Geometry check sheet. Reference: the model listing, model coordinates, mm. A direction names the side the tool comes from. Round coordinates to 2 decimals unless told otherwise and drop trailing zeros. Order: outer loops, then holes, each group sorted by start corner. A loop starts at its lowest first (then second) coordinate and runs counter-clockwise, first axis right, second up. Notation, with made-up numbers: (53, 22) -> (111, 22) arc R12 cw to (111, 37) -> close; hole circle Ø9 at (-4.75, 57.25). An arc over 180 degrees is marked (long way). Use a Markdown table: item, result. Add a question column.
Item 1: Sectioned sample at D-D, the plane x = -43. Record the cut outline in (y, z), and give its area (3 significant figures).
Item 2: Set-up check for faces 1 (the flat face through (-2, -28, -32.703)), 2 (the flat face through (-47.067, -29, 8)): record each of +Z, -Z, +X, -X, +Y, -Y from which the full face is reachable in a straight line by a thin tool's end or side.
Item 3: Gauge pin test, flat ends, axial feed: pin 1 Ø10 at (x, z) = (-10.5, -6.5) entering from +Y; pin 2 Ø2 at (x, z) = (1, 13) entering from -Y. Record the tip position at first contact, or that the pin passes through.
Item 4: Sectioned sample at B-B, the plane z = 6.5. Record the cut outline in (x, y), and give its area (3 significant figures).
Item 5: Mould release check, pull along Y, two halves, no side actions. Record for faces 3 (the flat face through (0, 0, 8)), 4 (the flat face through (-49.567, -28, 8)), 5 (the flat face through (0, -2.5, 8)), 6 (the cylindrical face through (-0.626, -25.635, 46.686)): pulls with the +Y half, pulls with the -Y half, needs draft (parallel to the pull), parting line crosses it, or undercut.
Item 6: Sectioned sample at A-A, the plane y = -18. Record the cut outline in (x, z).
Item 7: Material ranges on probe 1 along Z at (x, y) = (-16.5, -36); probe 2 along X at (y, z) = (-5.5, 13.5); probe 3 along Y at (x, z) = (-37, -23.5), recorded low to high. Write a range as [from, to].
Item 8: Sectioned sample at C-C, the plane x = -13.5. Record the cut outline in (y, z), and give its area (3 significant figures).
from build123d import *

# Parameters (mm, degrees)
F3_T     = -2.5
F5_D     = 30
F5_DEPTH = 12
F5_TIP   = 9.0129092854


with BuildPart() as f2:
    # F2: sweep along a path in F1
    with BuildLine(Plane.YZ) as f2_path:
        Line((0, 0), (-55.432960391, 0))
    # F0 (on Front) → F2 (sweep)
    with BuildSketch(Plane.XZ):
        Polygon((-49.567040056, 47.953914851), (-49.567040056, 42.0879907906), (-49.567040056, -32.7025167644), (47.8072650731, -32.7025167644), (47.8072650731, 47.953914851), align=None)
    sweep(path=f2_path.line)

    # F3
    f3_openings = [f2.faces().sort_by_distance(p)[0] for p in [
        (-0.879887, -55.43296, 7.625699),
    ]]
    offset(amount=F3_T, openings=f3_openings)

    # F5
    with Locations(Plane.XY.offset(47.953914851)):
        with Locations((0, -40.6215079129)):
            Hole(F5_D / 2, depth=F5_DEPTH)
            with Locations((0, 0, -(F5_DEPTH + F5_TIP / 2))):  # 118° drill point
                Cone(0, F5_D / 2, F5_TIP, mode=Mode.SUBTRACT)


solid = f2.part
Found:
| question | item | result |
|---|---|---|
| 1 | outline | (-55.43, -32.7) -> (0, -32.7) -> (0, 47.95) -> (-55.43, 47.95) -> (-55.43, 45.45) -> (-2.5, 45.45) -> (-2.5, -30.2) -> (-55.43, -30.2) -> close |
| 1 | area | 466 mm2 |
| 2 | face 1 | -Z, +X, -X, +Y, -Y |
| 2 | face 2 | -Y |
| 3 | pin 1 | stops at y = 0 |
| 3 | pin 2 | stops at y = -2.5 |
| 4 | outline | (-49.57, -55.43) -> (-47.07, -55.43) -> (-47.07, -2.5) -> (45.31, -2.5) -> (45.31, -55.43) -> (47.81, -55.43) -> (47.81, 0) -> (-49.57, 0) -> close |
| 4 | area | 508 mm2 |
| 5 | face 3 | pulls with the +Y half |
| 5 | face 4 | needs draft |
| 5 | face 5 | pulls with the -Y half |
| 5 | face 6 | undercut |
| 6 | outline | (-49.57, -32.7) -> (47.81, -32.7) -> (47.81, 47.95) -> (-49.57, 47.95) -> close; hole (-47.07, -30.2) -> (45.31, -30.2) -> (45.31, 45.45) -> (-47.07, 45.45) -> close |
| 7 | probe 1 | z = [-32.7, -30.2], [45.45, 47.95] |
| 7 | probe 2 | x = [-49.57, -47.07], [45.31, 47.81] |
| 7 | probe 3 | y = [-2.5, 0] |
| 8 | outline | (-55.43, -32.7) -> (0, -32.7) -> (0, 47.95) -> (-34.08, 47.95) -> (-34.08, 45.45) -> (-2.5, 45.45) -> (-2.5, -30.2) -> (-55.43, -30.2) -> close; (-55.43, 45.45) -> (-47.16, 45.45) -> (-47.16, 47.95) -> (-55.43, 47.95) -> close |
| 8 | area | 434 mm2 |
